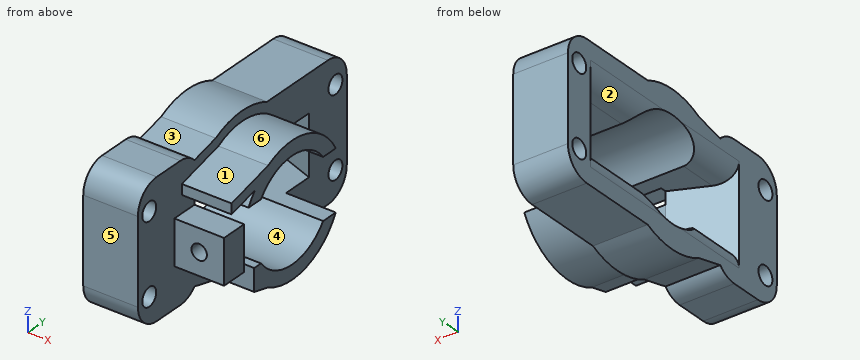
```python
from build123d import *

# Parameters (mm, degrees)
CROQUIS1_R              = 10
SALIENTE_EXTRUIR1_DEPTH = 11
CROQUIS2_R              = 10
SALIENTE_EXTRUIR2_DEPTH = 10
CORTAR_EXTRUIR3_DEPTH   = 10
CROQUIS8_R              = 1.55
CORTAR_EXTRUIR4_DEPTH   = 5
CORTAR_EXTRUIR5_REACH   = 52.656
CORTAR_EXTRUIR6_START   = -10
CORTAR_EXTRUIR6_DEPTH   = 10
SALIENTE_EXTRUIR5_DEPTH = 11
CORTAR_EXTRUIR9_REACH   = 59.413
CROQUIS19_R             = 1.85
SALIENTE_EXTRUIR7_DEPTH = 11
CROQUIS22_W             = 11
CROQUIS22_H             = 5
CORTAR_EXTRUIR10_DEPTH  = 12
CORTAR_EXTRUIR11_DEPTH  = 12
REDONDEO1_R             = 4
REDONDEO2_R             = 5
REDONDEO3_R             = 5


with BuildPart() as part:
    # Croquis1 → Saliente-Extruir1 (new body)
    with BuildSketch(Plane(origin=(0, 0, 0), x_dir=(0, 0, -1), z_dir=(1, 0, 0))):
        with BuildLine():
            Line((-5.780776406, 0), (-24.219223594, 0))
            ThreePointArc((-24.219223594, 0), (-24.834635803, 0.211794562), (-25.189366094, 0.757464375))
            Line((-25.189366094, 0.757464375), (-28.235294118, 12.941176471))
            ThreePointArc((-28.235294118, 12.941176471), (-15, 35), (-1.764705882, 12.941176471))
            Line((-1.764705882, 12.941176471), (-4.810633906, 0.757464375))
            ThreePointArc((-4.810633906, 0.757464375), (-5.165364197, 0.211794562), (-5.780776406, 0))
        make_face()
        with Locations((-15, 20)):
            Circle(CROQUIS1_R, mode=Mode.SUBTRACT)
    extrude(amount=SALIENTE_EXTRUIR1_DEPTH)

    # Croquis2 → Saliente-Extruir2 (add)
    with BuildSketch(Plane(origin=(11, 0, 0), x_dir=(0, 0, -1), z_dir=(1, 0, 0))):
        with BuildLine():
            Line((-23.477486008, 1.95), (-6.522513992, 1.95))
            Line((-6.522513992, 1.95), (-3.59620246, 13.655246131))
            ThreePointArc((-3.59620246, 13.655246131), (-15, 33.05), (-26.40379754, 13.655246131))
            Line((-26.40379754, 13.655246131), (-23.477486008, 1.95))
        make_face()
        with Locations((-15, 20)):
            Circle(CROQUIS2_R, mode=Mode.SUBTRACT)
    extrude(amount=SALIENTE_EXTRUIR2_DEPTH)

    # Croquis3 → Cortar-Extruir3 (cut)
    with BuildSketch(Plane(origin=(21, 0, 0), x_dir=(0, 0, -1), z_dir=(1, 0, 0))):
        Polygon((-9.522513992, 1.95), (-9.522513992, 9.95), (-4.522513992, 9.95), (-6.522513992, 1.95), align=None)
        with BuildLine():
            Line((-23.477486008, 1.95), (-18.477486008, 1.95))
            Line((-18.477486008, 1.95), (-18.477486008, 6.945227656))
            Line((-18.477486008, 6.945227656), (-18.477486008, 7.473743933))
            ThreePointArc((-18.477486008, 7.473743933), (-21.115240601, 8.528128645), (-23.461002355, 10.130276643))
            Line((-23.461002355, 10.130276643), (-23.242071918, 9.254554893))
            Line((-23.242071918, 9.254554893), (-21.915933195, 3.95))
            Line((-21.915933195, 3.95), (-23.977486008, 3.95))
            Line((-23.977486008, 3.95), (-23.477486008, 1.95))
        make_face()
    extrude(amount=-CORTAR_EXTRUIR3_DEPTH, mode=Mode.SUBTRACT)

    # Croquis8 → Cortar-Extruir4 (cut)
    with BuildSketch(Plane.XZ.offset(-1.95)):
        with Locations(Location((16, 14, 0), (0, 0, 270))):
            Circle(CROQUIS8_R)
    extrude(amount=-CORTAR_EXTRUIR4_DEPTH, mode=Mode.SUBTRACT)

    # Cortar-Extruir5: up to this face of the body (flat: up to its plane)
    cortar_extruir5_end = Plane(part.part.faces().sort_by_distance((21, 32.643992611, 15))[0])
    # Croquis11 → Cortar-Extruir5 (cut, up to the picked face)
    with BuildSketch(Plane.ZY, mode=Mode.PRIVATE) as cortar_extruir5_sk1:
        with BuildLine():
            Line((21, 32.7), (9, 32.7))
            Line((9, 32.7), (9, 28.248636251))
            ThreePointArc((9, 28.248636251), (4.8, 20), (9, 11.751363749))
            Line((9, 11.751363749), (9, 7.3))
            Line((9, 7.3), (21, 7.3))
            Line((21, 7.3), (21, 11.751363749))
            ThreePointArc((21, 11.751363749), (25.2, 20), (21, 28.248636251))
            Line((21, 28.248636251), (21, 32.7))
        make_face()
    cortar_extruir5_tool1 = split(extrude(cortar_extruir5_sk1.sketch, amount=-CORTAR_EXTRUIR5_REACH, mode=Mode.PRIVATE), bisect_by=cortar_extruir5_end, keep=Keep.BOTH, mode=Mode.PRIVATE)
    add(cortar_extruir5_tool1.solids().sort_by(Axis((0, 20, 15), (1, 0, 0)))[0], mode=Mode.SUBTRACT)

    # Croquis12 → Cortar-Extruir6 (cut)
    with BuildSketch(Plane(origin=(21, 0, 0), x_dir=(0, 0, -1), z_dir=(1, 0, 0)).offset(CORTAR_EXTRUIR6_START)):
        with BuildLine():
            Line((-18.00208261, 32.7), (-11.99791739, 32.7))
            ThreePointArc((-11.99791739, 32.7), (-15, 33.05), (-18.00208261, 32.7))
        make_face()
    extrude(amount=CORTAR_EXTRUIR6_DEPTH, mode=Mode.SUBTRACT)

    # Croquis18 → Saliente-Extruir5 (add)
    with BuildSketch(Plane.ZY):
        with BuildLine():
            Line((1.5, 7.3), (3.175, 7.3))
            Line((3.175, 7.3), (4.810633906, 0.757464375))
            ThreePointArc((4.810633906, 0.757464375), (5.165364197, 0.211794562), (5.780776406, 0))
            Line((5.780776406, 0), (24.219223594, 0))
            ThreePointArc((24.219223594, 0), (24.834635803, 0.211794562), (25.189366094, 0.757464375))
            Line((25.189366094, 0.757464375), (26.825, 7.3))
            Line((26.825, 7.3), (28.5, 7.3))
            Line((28.5, 7.3), (28.5, -7.7))
            Line((28.5, -7.7), (1.5, -7.7))
            Line((1.5, -7.7), (1.5, 7.3))
        make_face()
        with BuildLine():
            Line((1.5, 47.7), (28.5, 47.7))
            Line((28.5, 47.7), (28.5, 32.7))
            Line((28.5, 32.7), (22.981854421, 32.7))
            ThreePointArc((22.981854421, 32.7), (15, 35), (7.018145579, 32.7))
            Line((7.018145579, 32.7), (1.5, 32.7))
            Line((1.5, 32.7), (1.5, 47.7))
        make_face()
    extrude(amount=-SALIENTE_EXTRUIR5_DEPTH)

    # Croquis19 → Cortar-Extruir9 (cut, up to next)
    with BuildSketch(Plane(origin=(11, 0, 0), x_dir=(0, 0, -1), z_dir=(1, 0, 0)), mode=Mode.PRIVATE) as cortar_extruir9_sk1:
        with Locations((-23, -4.7)):
            Circle(CROQUIS19_R)
    cortar_extruir9_tool1 = extrude(cortar_extruir9_sk1.sketch, amount=-CORTAR_EXTRUIR9_REACH, mode=Mode.PRIVATE) & part.part
    # Croquis19 → Cortar-Extruir9 (cut, up to next)
    with BuildSketch(Plane(origin=(11, 0, 0), x_dir=(0, 0, -1), z_dir=(1, 0, 0)), mode=Mode.PRIVATE) as cortar_extruir9_sk2:
        with Locations(Location((-7, -4.7, 0), (0, 0, 180))):
            Circle(CROQUIS19_R)
    cortar_extruir9_tool2 = extrude(cortar_extruir9_sk2.sketch, amount=-CORTAR_EXTRUIR9_REACH, mode=Mode.PRIVATE) & part.part
    # Croquis19 → Cortar-Extruir9 (cut, up to next)
    with BuildSketch(Plane(origin=(11, 0, 0), x_dir=(0, 0, -1), z_dir=(1, 0, 0)), mode=Mode.PRIVATE) as cortar_extruir9_sk3:
        with Locations((-7, 44.7)):
            Circle(CROQUIS19_R)
    cortar_extruir9_tool3 = extrude(cortar_extruir9_sk3.sketch, amount=-CORTAR_EXTRUIR9_REACH, mode=Mode.PRIVATE) & part.part
    # Croquis19 → Cortar-Extruir9 (cut, up to next)
    with BuildSketch(Plane(origin=(11, 0, 0), x_dir=(0, 0, -1), z_dir=(1, 0, 0)), mode=Mode.PRIVATE) as cortar_extruir9_sk4:
        with Locations(Location((-23, 44.7, 0), (0, 0, 180))):
            Circle(CROQUIS19_R)
    cortar_extruir9_tool4 = extrude(cortar_extruir9_sk4.sketch, amount=-CORTAR_EXTRUIR9_REACH, mode=Mode.PRIVATE) & part.part
    add(cortar_extruir9_tool1.solids().sort_by_distance((11, -4.7, 23))[0], mode=Mode.SUBTRACT)
    add(cortar_extruir9_tool2.solids().sort_by_distance((11, -4.7, 7))[0], mode=Mode.SUBTRACT)
    add(cortar_extruir9_tool3.solids().sort_by_distance((11, 44.7, 7))[0], mode=Mode.SUBTRACT)
    add(cortar_extruir9_tool4.solids().sort_by_distance((11, 44.7, 23))[0], mode=Mode.SUBTRACT)

    # Croquis21 → Saliente-Extruir7 (add)
    with BuildSketch(Plane.ZY):
        with BuildLine():
            Line((22.981854421, 32.7), (28.5, 32.7))
            Line((28.5, 32.7), (28.5, 26.538348415))
            ThreePointArc((28.5, 26.538348415), (26.174032616, 30.007047272), (22.981854421, 32.7))
        make_face()
        with BuildLine():
            Line((1.5, 32.7), (7.018145579, 32.7))
            ThreePointArc((7.018145579, 32.7), (3.825967384, 30.007047272), (1.5, 26.538348415))
            Line((1.5, 26.538348415), (1.5, 32.7))
        make_face()
    extrude(amount=-SALIENTE_EXTRUIR7_DEPTH)

    # Croquis22 → Cortar-Extruir10 (cut)
    with BuildSketch(Plane.XY.offset(9)):
        Polygon((0, 7.3), (0, 2.3), (11, 7.3), align=None)
        with Locations((5.5, 35.2)):
            Rectangle(CROQUIS22_W, CROQUIS22_H)
    extrude(amount=CORTAR_EXTRUIR10_DEPTH, mode=Mode.SUBTRACT)

    # Croquis23 → Cortar-Extruir11 (cut)
    with BuildSketch(Plane.XY.offset(9)):
        Polygon((0, 37.7), (11, 37.7), (0, 41.7), align=None)
    extrude(amount=CORTAR_EXTRUIR11_DEPTH, mode=Mode.SUBTRACT)

    # Redondeo1
    redondeo1_edges = [part.edges().sort_by_distance(p)[0] for p in [
        (0, 34.974318125, 21),
        (0, 34.974318125, 9),
        (0, 7.025681875, 9),
        (0, 7.025681875, 21),
    ]]
    fillet(redondeo1_edges, radius=REDONDEO1_R)

    # Redondeo2
    # the kernel refuses this fillet: 5 mm, written as the material it takes off along each edge
    with BuildSketch(Plane(origin=(-9.335541963, 7.3, 28.5), x_dir=(0, 0, -1), z_dir=(1, 0, 0))) as redondeo2_piece_1:
        with BuildLine():
            CenterArc((5, -3.734216785), REDONDEO2_R, 131.682325393, 48.317674607)
            Line((0, -3.734216785), (-0.1, -3.734216785))
            Line((-0.1, -3.734216785), (-0.1, 0))
            Line((-0.1, 0), (0, 0.1))
            ThreePointArc((0, 0.1), (0.8375, 0.1), (1.6085, 0.074684336))
            Line((1.6085, 0.074684336), (1.675, 0))
        make_face()
    extrude(amount=29.671083927, mode=Mode.SUBTRACT)
    with BuildSketch(Plane(origin=(-9.335541963, 7.3, 1.5), x_dir=(0, -1, 0), z_dir=(1, 0, 0))) as redondeo2_piece_2:
        with BuildLine():
            CenterArc((3.734216785, -5), REDONDEO2_R, 90, 48.317674607)
            Line((0, -1.675), (-0.074684336, -1.6085))
            ThreePointArc((-0.074684336, -1.6085), (-0.1, -0.8375), (-0.1, 0))
            Line((-0.1, 0), (0, 0.1))
            Line((0, 0.1), (3.734216785, 0.1))
            Line((3.734216785, 0.1), (3.734216785, 0))
        make_face()
    extrude(amount=29.671083927, mode=Mode.SUBTRACT)

    # Redondeo3
    redondeo3_edges = [part.edges().sort_by_distance(p)[0] for p in [
        (5.5, -7.7, 1.5),
        (5.5, -7.7, 28.5),
        (5.5, 47.7, 1.5),
        (5.5, 47.7, 28.5),
    ]]
    fillet(redondeo3_edges, radius=REDONDEO3_R)


solid = part.part
```
Could you check a few things on this model? Use its own coordinates, in mm. Face numbers are marked on the shaded views. A direction names the side the tool comes from. Coordinates: 2 decimals unless noted, no trailing zeros. Loops run counter-clockwise (first coordinate to the right, second up) from the corner with the lowest first, then second, coordinate; pieces in that order, holes last. Notation, with made-up numbers: M -31,11.25 L 2,11.25 A4 cw 2,15.25 Z; hole C -26,-3.75 d4. An arc over 180 degrees is marked long. Put each result on its own line as item: value. Start each with the question number.
(1) For the marked faces 1, 2 and 3, which set-ups out of +Z, -Z, +X, -X, +Y, -Y let a thin tool reach every point of the face, with its end or its side?
(2) Suppose I cut it at B-B on z = 14. Please give me the cut outline in (x, y).
(3) I need wall thicknesses on line 1 (Z direction, x = 18, y = 19.5); line 2 (X direction, y = 44, z = 16.5); line 3 (Z direction, x = 3.25, y = 31). Which ranges of each line are inside material? Lowest first, please. Write a range as from..to.
(4) Suppose I cut it at C-C on y = 37. Please give me the cut outline in (x, z).
(5) Suppose I cut it at A-A on x = 16. Please give me the cut outline in (y, z).
(6) Suppose I cut it at D-D on x = 10. Please give me the cut outline in (y, z) (3 decimals), then the cut area to 3 significant figures.
(7) Will these pins go through, and if not, where does the flat tip stop? P1, Ø9, axis at x = 7, y = 37, coming from the +Z side; P2, Ø1, axis at x = 14, z = 23.5, coming from the -Y side; P3, Ø4, axis at y = 36.5, z = 22, coming from the +X side; P4, Ø3, axis at y = 44.7, z = 23, coming from the +X side.
(8) Thinking about a two-plate mould opening in Y: for the marked faces 4, 5 and 6, which applies, pulls with the +Y half, pulls with the -Y half, needs draft (parallel to the pull), parting line crosses it, or undercut?
Solutions:
1. face 1: +Z, +X, -Y
1. face 2: -X
1. face 3: +Z, +X, -X
2. outline: M 0,-7.7 L 11,-7.7 L 11,1.95 L 14.45,1.95 L 14.45,6.95 L 17.55,6.95 L 17.55,1.95 L 21,1.95 L 21,7.3 L 11,7.3 L 0,2.3 Z; M 0,41.7 L 11,37.7 L 11,47.7 L 0,47.7 Z
3. line 1: z = 1.96..4.81, 25.19..28.04
3. line 2: x = 0..11
3. line 3: z = 1.5..8.93, 21.07..28.5
4. outline: M 0,1.5 L 11,1.5 L 11,9 L 4,9 A4 ccw 0,5 Z; M 0,25 A4 ccw 4,21 L 11,21 L 11,28.5 L 0,28.5 Z
5. outline: M 1.95,9.52 L 7.3,9.52 L 7.3,18.48 L 1.95,18.48 L 1.95,15.55 L 6.95,15.55 L 6.95,12.45 L 1.95,12.45 Z; M 3.95,21.92 L 10.13,23.46 A13 ccw 8.47,21 L 11.75,21 A10.2 cw 28.25,21 L 31.59,21 A13.05 ccw 13.66,26.4 L 3.95,23.98 Z; M 9.95,4.52 L 13.66,3.6 A13.05 ccw 31.59,9 L 28.25,9 A10.2 cw 11.75,9 L 9.95,9 Z
6. outline: M -7.7,6.5 A5 ccw -2.7,1.5 L 3.566,1.5 A5 ccw 7.3,3.175 L 12.941,1.765 A15 ccw 26.538,1.5 L 42.7,1.5 A5 ccw 47.7,6.5 L 47.7,23.5 A5 ccw 42.7,28.5 L 26.538,28.5 A15 ccw 12.941,28.235 L 7.3,26.825 A5 ccw 3.566,28.5 L -2.7,28.5 A5 ccw -7.7,23.5 Z; hole C -4.7,7 d3.7; hole C -4.7,23 d3.7; hole M 6.845,9 L 11.751,9 A10.2 ccw 28.249,9 L 38.064,9 L 38.064,21 L 28.249,21 A10.2 ccw 11.751,21 L 6.845,21 Z; hole C 44.7,7 d3.7; hole C 44.7,23 d3.7
6. area: 971 mm2
7. P1: stops at z = 28.5
7. P2: stops at y = 3.95
7. P3: stops at x = 11
7. P4: passes through
8. face 4: undercut
8. face 5: pulls with the -Y half
8. face 6: parting line crosses it
